from build123d import *

# Parameters (mm, degrees)
BOSS_EXTRU_1_DEPTH = 2
BOSS_EXTRU_2_START = 2
BOSS_EXTRU_2_DEPTH = 4
CONG_1_R           = 9


with BuildPart() as part:
    # Esquisse1 → Boss.-Extru.1 (new body)
    with BuildSketch(Plane.XY):
        Polygon((-40.70550554, -19.868421053), (-30.70550554, -19.868421053), (-30.70550554, 130.131578947), (169.29449446, 130.131578947), (169.29449446, -19.868421053), (179.29449446, -19.868421053), (179.29449446, 140.131578947), (-40.70550554, 140.131578947), align=None)
    extrude(amount=BOSS_EXTRU_1_DEPTH)

    # Esquisse2 → Boss.-Extru.2 (add)
    with BuildSketch(Plane.XY.offset(BOSS_EXTRU_2_START)):
        Polygon((-30.70550554, -19.868421053), (-28.70550554, -19.868421053), (-28.70550554, 128.131578947), (167.29449446, 128.131578947), (167.29449446, -19.868421053), (169.29449446, -19.868421053), (169.29449446, 130.131578947), (-30.70550554, 130.131578947), align=None)
    extrude(amount=-BOSS_EXTRU_2_DEPTH)

    # Congé1
    cong_1_edges = [part.edges().sort_by_distance(p)[0] for p in [
        (-40.70550554, 140.131578947, 1),
        (179.29449446, 140.131578947, 1),
        (179.29449446, -19.868421053, 1),
        (-40.70550554, -19.868421053, 1),
    ]]
    fillet(cong_1_edges, radius=CONG_1_R)


solid = part.part
Can you work these out from the model? Positions are in its coordinate system, mm. Give positions to 0.01 mm unless a question says otherwise; leave off trailing zeros. Order: outer loops, then holes, each group sorted by start corner. A loop starts at its lowest first (then second) coordinate and runs counter-clockwise, first axis right, second up. Notation, with made-up numbers: M -14,-28 L 23,-28 A28 ccw 23,1 Z; hole C 5,16.25 d6. An arc over 180 degrees is marked long. Use one line per item in the form item = value. Start each with the question number.
Item 1: Will these pins go through, and if not, where does the flat tip stop? pin 1 Ø1.5 at (x, z) = (134.5, -1) entering from -Y; pin 2 Ø0.6 at (y, z) = (28.5, -1) entering from -X; pin 3 Ø1.5 at (x, z) = (151.5, -1.5) entering from +Y.
Item 2: If we section it at A-A (y = 110.5): Write out the boundary of the cut face in (x, z).
Item 3: If I drill on line 1 along X through (y, z) = (16, -1.35); line 2 along X through (y, z) = (48, 1.15); line 3 along Y through (x, z) = (77, 0.65), over which ranges is the centre line in solid material (lowest first)?
Item 4: If we section it at B-B (z = -0.8): Write out the boundary of the cut face in (x, y).
Item 5: If we section it at C-C (x = 47): Write out the boundary of the cut face in (y, z).
Outcome:
q1.pin_1 = 128.13
q1.pin_2 = -30.71
q1.pin_3 = 130.13
q2.outline = M -40.71,0 L -30.71,0 L -30.71,-2 L -28.71,-2 L -28.71,2 L -40.71,2 Z; M 167.29,-2 L 169.29,-2 L 169.29,0 L 179.29,0 L 179.29,2 L 167.29,2 Z
q3.line_1 = -30.71 to -28.71, 167.29 to 169.29
q3.line_2 = -40.71 to -28.71, 167.29 to 179.29
q3.line_3 = 128.13 to 140.13
q4.outline = M -30.71,-19.87 L -28.71,-19.87 L -28.71,128.13 L 167.29,128.13 L 167.29,-19.87 L 169.29,-19.87 L 169.29,130.13 L -30.71,130.13 Z
q5.outline = M 128.13,-2 L 130.13,-2 L 130.13,0 L 140.13,0 L 140.13,2 L 128.13,2 Z
